Source: CAD feature listing. Evaluate the final solid. Frame: model axes, mm. Give positions to 0.01 mm unless a question says otherwise; leave off trailing zeros. Order: outer loops, then holes, each group sorted by start corner. A loop starts at its lowest first (then second) coordinate and runs counter-clockwise, first axis right, second up. Notation, with made-up numbers: (1, 2) -> (45, 2) arc R18 cw to (45, 34) -> close; hole circle Ø6 at (55, 74). An arc over 180 degrees is marked (long way). Answer in a Markdown table with one row per item.
Autodesk Inventor part; units mm, degrees
ref_plane "YZ Plane" through (0, 0, 0) normal (1, 0, 0) x (0, 1, 0)
ref_plane "XZ Plane" through (0, 0, 0) normal (0, 1, 0) x (-1, 0, 0)
ref_plane "XY Plane" through (0, 0, 0) normal (0, 0, 1) x (1, 0, 0)
sketch "Sketch1" plane through (0, 0, 0) normal (0, 0, 1) x (1, 0, 0)
  line L0 (-571.5, -609.6) -> (571.5, -609.6)
  line L1 (571.5, -609.6) -> (571.5, 609.6)
  line L2 (571.5, 609.6) -> (-571.5, 609.6)
  line L3 (-571.5, 609.6) -> (-571.5, -609.6)
  line L4 (-571.5, -609.6) -> (571.5, 609.6) construction
  line L5 (571.5, -609.6) -> (-571.5, 609.6) construction
  line L6 (571.5, 609.6) -> (-571.5, -609.6)
  line L7 (-539.0721, -640.0012) -> (-603.9279, -579.1988)
  line L8 (603.9279, 579.1988) -> (539.0721, 640.0012)
  line L9 (539.0721, 640.0012) -> (-603.9279, -579.1988)
  line L10 (603.9279, 579.1988) -> (-539.0721, -640.0012)
  point P0 (0, 0)
  point P1 (510.571, 609.6)
  point P2 (-571.5, -544.609)
  point P3 (-510.571, -609.6)
  point P4 (571.5, 544.609)
  dimension "d0" = 1143
  dimension "d1" = 1219.2
  dimension "d2" = 88.9
  dimension "d3" = 88.9
extrude "Extrusion1" add sketch "Sketch1" along normal blind 38.1 contours L6 L1 L10 L0 | L3 L9 L2 L6
properties part number "S_2x4x65.795"
(1) Section query A-A (z = 20). Return the cut outline in (x, y), plus the area to 3 significant figures.
A:
| item | result |
|---|---|
| outline | (-571.5, -609.6) -> (-510.57, -609.6) -> (571.5, 544.61) -> (571.5, 609.6) -> (510.57, 609.6) -> (-571.5, -544.61) -> close |
| area | 145,000 mm^2 |
(2) Section query B-B (y = 51). Return the cut outline in (x, z).
A:
| item | result |
|---|---|
| outline | (-13.12, 0) -> (108.74, 0) -> (108.74, 38.1) -> (-13.12, 38.1) -> close |
(3) Section query C-C (x = 324). Return the cut outline in (y, z), plus the area to 3 significant figures.
A:
| item | result |
|---|---|
| outline | (280.61, 0) -> (410.59, 0) -> (410.59, 38.1) -> (280.61, 38.1) -> close |
| area | 4,950 mm^2 |
(4) Ray query, probe 1 along X at (y, z) = (447, 4); probe 2 along X at (y, z) = (-496.5, 21); probe 3 along Y at (x, z) = (153.5, 8.5). Return the intervals inside material, ascending.
A:
| item | result |
|---|---|
| probe 1 | x = 358.13 to 479.99 |
| probe 2 | x = -526.4 to -404.54 |
| probe 3 | y = 98.74 to 228.72 |
(5) First-contact query: pin 1 Ø2 at (x, z) = (3.5, 8) entering from +Y; pin 2 Ø12 at (y, z) = (-171, 4) entering from -X; pin 3 Ø5 at (x, z) = (-159.5, 4.5) entering from +Y. Flat tips, straight axial feed; report the tip coordinate or a pass-through.
A:
| item | result |
|---|---|
| pin 1 | stops at y = 69.79 |
| pin 2 | stops at x = -226.87 |
| pin 3 | stops at y = -102.48 |
